Read the model definition and answer for the solid it produces. Units are mm, in the model's axes. Face numbers are marked on the shaded views. A direction names the side the tool comes from. Coordinates: 2 decimals unless noted, no trailing zeros. Write each loop counter-clockwise with the first axis right and the second up, starting at its lowest first coordinate (ties: lowest second). Pieces come first, ordered by that corner, then holes.
Item 1: A tool of negligible diameter and unlimited length cuts with its end or side. For the marked faces 4, 5, 6, 7 and 8, from which of +Z, -Z, +X, -X, +Y, -Y can it reach the whole face along a straight path? Write none if from no direction.
Item 2: Each of these flat-tipped pins is pushed along its axis until it touches: P1, Ø4, axis at y = 2.5, z = 35, coming from the +X side; P2, Ø4.5, axis at x = 3.5, y = -0.5, coming from the +Z side; P3, Ø6, axis at y = -1, z = 8.5, coming from the +X side. Where does it stop, or does it pass through?
Item 3: Section D-D (x = -2) is taken. Give the vertices of the cut face in (y, z), then the cut area to 3 significant figures.
Item 4: Straight lines are drawn through the part: probe 1 along X at (y, z) = (0.25, 18); probe 2 along Z at (x, y) = (24, 0); probe 3 along Y at (x, z) = (5, 10). For each, find the intervals that lie inside material, in ascending order.
Item 5: Section A-A (x = 27) is taken. Give the vertices of the cut face in (y, z), then the cut area to 3 significant figures.
Item 6: Section B-B (y = 0) is taken. State how many separate pieces and enclosed holes the cut face has, then the cut area to 3 significant figures.
Item 7: Determine the mould class of the marked faces 1, 2 and 3 for opening direction X: released by +X, released by -X, zero draft, split by the parting line, or undercut.
Item 8: Section C-C (z = 29) is taken. Give the vertices of the cut face in (x, y), then the cut area to 3 significant figures.
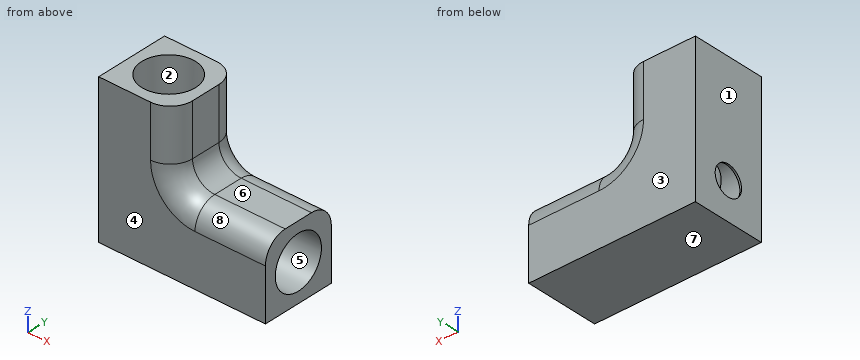
from build123d import *

# Parameters (mm, degrees)
SKETCH_2_W                 = 20
SKETCH_2_H                 = 20
EXTRUDE_482_DEPTH          = 40
SKETCH_4_W                 = 20
SKETCH_4_H                 = 20
EXTRUDE_639_DEPTH          = 25
SKETCH_7_R                 = 6
CUT_EXTRUDE_822_DEPTH      = 44
CUT_EXTRUDE_968_REACH      = 56.083
CUT_EXTRUDE_968_END_RADIUS = 6
SKETCH_8_R                 = 6
SKETCH_9_R                 = 7.25
CUT_EXTRUDE_1104_DEPTH     = 20
SKETCH_10_R                = 7
CUT_EXTRUDE_1247_DEPTH     = 20
CUT_EXTRUDE_1380_REACH     = 63.033
SKETCH_11_R                = 4
FILLET_2_R                 = 6
FILLET_5_R                 = 1


with BuildPart() as part:
    # Эскиз2 → Extrude 482 (new body)
    with BuildSketch(Plane.XY):
        Rectangle(SKETCH_2_W, SKETCH_2_H)
    extrude(amount=EXTRUDE_482_DEPTH)

    # Эскиз4 → Extrude 639 (add)
    with BuildSketch(Plane(origin=(10, 0, 0), x_dir=(0, 0, -1), z_dir=(1, 0, 0))):
        with Locations((-10, 0)):
            Rectangle(SKETCH_4_W, SKETCH_4_H)
    extrude(amount=EXTRUDE_639_DEPTH)

    # Эскиз7 → Cut-Extrude 822 (cut)
    with BuildSketch(Plane(origin=(35, 0, 0), x_dir=(0, 0, -1), z_dir=(1, 0, 0))):
        with Locations(Location((-10, 0, 0), (0, 0, 90))):
            Circle(SKETCH_7_R)
    extrude(amount=-CUT_EXTRUDE_822_DEPTH, mode=Mode.SUBTRACT)

    # Cut-Extrude 968: up to this cylinder (the profile starts outside it)
    cut_extrude_968_end = Plane(origin=(0, 0, 10), z_dir=(1, 0, 0)) * Cylinder(CUT_EXTRUDE_968_END_RADIUS, 125.166, mode=Mode.PRIVATE)
    # Эскиз8 → Cut-Extrude 968 (cut, up to the surface)
    with BuildSketch(Plane.XY.offset(40), mode=Mode.PRIVATE) as cut_extrude_968_sk1:
        Circle(SKETCH_8_R)
    cut_extrude_968_tool1 = extrude(cut_extrude_968_sk1.sketch, amount=-CUT_EXTRUDE_968_REACH, mode=Mode.PRIVATE) - cut_extrude_968_end
    add(cut_extrude_968_tool1.solids().sort_by_distance((0, 0, 40))[0], mode=Mode.SUBTRACT)

    # Эскиз9 → Cut-Extrude 1104 (cut)
    with BuildSketch(Plane.XY.offset(40)):
        Circle(SKETCH_9_R)
    extrude(amount=-CUT_EXTRUDE_1104_DEPTH, mode=Mode.SUBTRACT)

    # Эскиз10 → Cut-Extrude 1247 (cut)
    with BuildSketch(Plane(origin=(35, 0, 0), x_dir=(0, 0, -1), z_dir=(1, 0, 0))):
        with Locations(Location((-10, 0, 0), (0, 0, 90))):
            Circle(SKETCH_10_R)
    extrude(amount=-CUT_EXTRUDE_1247_DEPTH, mode=Mode.SUBTRACT)

    # Эскиз11 → Cut-Extrude 1380 (cut, up to next)
    with BuildSketch(Plane.ZY.offset(10), mode=Mode.PRIVATE) as cut_extrude_1380_sk1:
        with Locations(Location((10, 0, 0), (0, 0, 270))):
            Circle(SKETCH_11_R)
    cut_extrude_1380_tool1 = extrude(cut_extrude_1380_sk1.sketch, amount=-CUT_EXTRUDE_1380_REACH, mode=Mode.PRIVATE) & part.part
    add(cut_extrude_1380_tool1.solids().sort_by_distance((-10, 0, 10))[0], mode=Mode.SUBTRACT)

    # Скругление2
    fillet_2_edges = [part.edges().sort_by_distance(p)[0] for p in [
        (10, 0, 20),
        (22.5, 10, 20),
        (22.5, -10, 20),
        (10, -10, 30),
        (10, 10, 30),
    ]]
    fillet(fillet_2_edges, radius=FILLET_2_R)

    # Скругление5
    fillet_5_edges = [part.edges().sort_by_distance(p)[0] for p in [
        (-9, 4, 10),
    ]]
    fillet(fillet_5_edges, radius=FILLET_5_R - 0.0001)  # a hair under: the kernel refuses the full size


solid = part.part
Established:
1. face 4: +Z, -Z, +X, -X, -Y
1. face 5: +X
1. face 6: +Z, +X, +Y, -Y
1. face 7: -Z, +X, -X, +Y, -Y
1. face 8: +Z, +X, -Y
2. P1: stops at x = 10
2. P2: stops at z = 4.67
2. P3: stops at x = -9.02
3. outline: (-10, 0) - (10, 0) - (10, 40) - (6.97, 40) - (6.97, 20) - (5.66, 20) - (5.66, 12) arc R6 cw (long way) to (-5.66, 12) - (-5.66, 20) - (-6.97, 20) - (-6.97, 40) - (-10, 40) - close
3. area: 351 mm2
4. probe 1: x = -10 to -5.99, 5.99 to 35
4. probe 2: z = 0 to 3, 17 to 20
4. probe 3: y = -10 to -6, 6 to 10
5. outline: (-10, 0) - (10, 0) - (10, 14) arc R6 ccw to (4, 20) - (-4, 20) arc R6 ccw to (-10, 14) - close; hole circle Ø14 at (0, 10)
5. area: 231 mm2
6. separate pieces: 3
6. enclosed holes: 0
6. area: 393 mm2
7. face 1: released by -X
7. face 2: undercut
7. face 3: zero draft
8. outline: (-10, -10) - (4, -10) arc R6 ccw to (10, -4) - (10, 4) arc R6 ccw to (4, 10) - (-10, 10) - close; hole circle Ø14.5 at (0, 0)
8. area: 219 mm2
